```python
from build123d import *

# Parameters (mm, degrees)
SKETCH1_W                          = 200
SKETCH1_H                          = 90
BOSS_EXTRUDE1_DEPTH                = 40
SHAFTFITS_WITH_5MM_TOLERANCE_REACH = 120.743
SKETCH2_R                          = 3
SHAFTFITTOLERANCE_DEPTH            = 40
SKETCH3_R                          = 8.075
PULLEY_DEPTH                       = 30
SKETCH4_R                          = 26.5
GEARS_FITS_DEPTH                   = 10
GEAR_LETOUT_REACH                  = 120.743
SKETCH5_W                          = 200
SKETCH5_H                          = 30
CLOSED_LOOP_TIMING_BELT_REACH      = 116.891
SKETCH8_W                          = 60
SKETCH8_H                          = 3
SKETCH7_R                          = 10.075
PULLEY_MARGIN_DEPTH                = 20
SKETCH6_R                          = 28.5
GEAR_MARGIN_DEPTH                  = 10
PULLEYFIXTOLERANCE_DEPTH           = 30
GEARFITSTOLERANCE_DEPTH            = 10
M3_SCREWHOLES_REACH                = 116.891
M3_SCREWHEADS_DEPTH                = 5
M3_SCREWHEADS_DIRECTION_2_REACH    = 113.803
SKETCH16_W                         = 33
SKETCH16_H                         = 60
REMOVEEXTRA1_DEPTH                 = 40
SKETCH17_W                         = 5
SKETCH17_H                         = 60
REMOVEEXTRA2_DEPTH                 = 40


with BuildPart() as part:
    # Sketch1 → Boss-Extrude1 (new body)
    with BuildSketch(Plane.XY):
        with Locations((0, -5)):
            Rectangle(SKETCH1_W, SKETCH1_H)
    extrude(amount=BOSS_EXTRUDE1_DEPTH)

    # Sketch2 → ShaftFits_with.5mm_tolerance (cut, up to next)
    with BuildSketch(Plane.XY.offset(40), mode=Mode.PRIVATE) as shaftfits_with_5mm_tolerance_sk1:
        with Locations((30, 0)):
            Circle(SKETCH2_R)
    shaftfits_with_5mm_tolerance_tool1 = extrude(shaftfits_with_5mm_tolerance_sk1.sketch, amount=-SHAFTFITS_WITH_5MM_TOLERANCE_REACH, mode=Mode.PRIVATE) & part.part
    # Sketch2 → ShaftFits_with.5mm_tolerance (cut, up to next)
    with BuildSketch(Plane.XY.offset(40), mode=Mode.PRIVATE) as shaftfits_with_5mm_tolerance_sk2:
        with Locations(Location((-30, 0, 0), (0, 0, 180))):
            Circle(SKETCH2_R)
    shaftfits_with_5mm_tolerance_tool2 = extrude(shaftfits_with_5mm_tolerance_sk2.sketch, amount=-SHAFTFITS_WITH_5MM_TOLERANCE_REACH, mode=Mode.PRIVATE) & part.part
    add(shaftfits_with_5mm_tolerance_tool1.solids().sort_by_distance((30, 0, 40))[0], mode=Mode.SUBTRACT)
    add(shaftfits_with_5mm_tolerance_tool2.solids().sort_by_distance((-30, 0, 40))[0], mode=Mode.SUBTRACT)

    # Sketch9 → ShaftFitTolerance (cut)
    with BuildSketch(Plane.XY.offset(40)):
        with BuildLine():
            Line((30, 3), (35, 3))
            ThreePointArc((35, 3), (38, 0), (35, -3))
            Line((35, -3), (30, -3))
            ThreePointArc((30, -3), (27, 0), (30, 3))
        make_face()
    extrude(amount=-SHAFTFITTOLERANCE_DEPTH, mode=Mode.SUBTRACT)

    # Sketch3 → Pulley (cut)
    with BuildSketch(Plane.XY.offset(40)):
        with Locations((30, 0)):
            Circle(SKETCH3_R)
        with Locations(Location((-30, 0, 0), (0, 0, 180))):
            Circle(SKETCH3_R)
    extrude(amount=-PULLEY_DEPTH, mode=Mode.SUBTRACT)

    # Sketch4 → Gears fits (cut)
    with BuildSketch(Plane.XY.offset(40)):
        with Locations((30, 0)):
            Circle(SKETCH4_R)
        with Locations(Location((-30, 0, 0), (0, 0, 180))):
            Circle(SKETCH4_R)
    extrude(amount=-GEARS_FITS_DEPTH, mode=Mode.SUBTRACT)

    # Sketch5 → Gear letout (cut, up to next)
    with BuildSketch(Plane.XY.offset(40), mode=Mode.PRIVATE) as gear_letout_sk1:
        with Locations((0, -35)):
            Rectangle(SKETCH5_W, SKETCH5_H)
    gear_letout_tool1 = extrude(gear_letout_sk1.sketch, amount=-GEAR_LETOUT_REACH, mode=Mode.PRIVATE) & part.part
    add(gear_letout_tool1.solids().sort_by_distance((0, -35, 40))[0], mode=Mode.SUBTRACT)

    # Closed-loop timing belt: up to this face of the body (flat: up to its plane)
    closed_loop_timing_belt_end = Plane(part.part.faces().sort_by_distance((-22.15339549, 0, 10))[0])
    # Sketch8 → Closed-loop timing belt (cut, up to the picked face)
    with BuildSketch(Plane.XY.offset(40), mode=Mode.PRIVATE) as closed_loop_timing_belt_sk1:
        with Locations((0, 6.575)):
            Rectangle(SKETCH8_W, SKETCH8_H)
    closed_loop_timing_belt_tool1 = split(extrude(closed_loop_timing_belt_sk1.sketch, amount=-CLOSED_LOOP_TIMING_BELT_REACH, mode=Mode.PRIVATE), bisect_by=closed_loop_timing_belt_end, keep=Keep.BOTH, mode=Mode.PRIVATE)
    # Sketch8 → Closed-loop timing belt (cut, up to the picked face)
    with BuildSketch(Plane.XY.offset(40), mode=Mode.PRIVATE) as closed_loop_timing_belt_sk2:
        with Locations((0, -6.575)):
            Rectangle(SKETCH8_W, SKETCH8_H)
    closed_loop_timing_belt_tool2 = split(extrude(closed_loop_timing_belt_sk2.sketch, amount=-CLOSED_LOOP_TIMING_BELT_REACH, mode=Mode.PRIVATE), bisect_by=closed_loop_timing_belt_end, keep=Keep.BOTH, mode=Mode.PRIVATE)
    add(closed_loop_timing_belt_tool1.solids().sort_by(Axis((0, 6.575, 40), (0, 0, -1)))[0], mode=Mode.SUBTRACT)
    add(closed_loop_timing_belt_tool2.solids().sort_by(Axis((0, -6.575, 40), (0, 0, -1)))[0], mode=Mode.SUBTRACT)

    # Sketch7 → Pulley margin (cut)
    with BuildSketch(Plane.XY.offset(30)):
        with Locations((30, 0)):
            Circle(SKETCH7_R)
        with Locations((-30, 0)):
            Circle(SKETCH7_R)
    extrude(amount=-PULLEY_MARGIN_DEPTH, mode=Mode.SUBTRACT)

    # Sketch6 → Gear margin (cut)
    with BuildSketch(Plane.XY.offset(40)):
        with Locations((30, 0)):
            Circle(SKETCH6_R)
        with Locations((-30, 0)):
            Circle(SKETCH6_R)
    extrude(amount=-GEAR_MARGIN_DEPTH, mode=Mode.SUBTRACT)

    # Sketch12 → PulleyFixTolerance (cut)
    with BuildSketch(Plane.XY.offset(40)):
        with BuildLine():
            Line((30, 10.075), (35, 10.075))
            ThreePointArc((35, 10.075), (45.075, 0), (35, -10.075))
            Line((35, -10.075), (30, -10.075))
            ThreePointArc((30, -10.075), (19.925, 0), (30, 10.075))
        make_face()
    extrude(amount=-PULLEYFIXTOLERANCE_DEPTH, mode=Mode.SUBTRACT)

    # Sketch13 → GearFitsTolerance (cut)
    with BuildSketch(Plane.XY.offset(40)):
        with BuildLine():
            Line((30, 28.5), (35, 28.5))
            ThreePointArc((35, 28.5), (63.5, 0), (35, -28.5))
            Line((35, -28.5), (30, -28.5))
            ThreePointArc((30, -28.5), (1.5, 0), (30, 28.5))
        make_face()
    extrude(amount=-GEARFITSTOLERANCE_DEPTH, mode=Mode.SUBTRACT)

    # M3 ScrewHoles: up to this face of the body (flat: up to its plane)
    m3_screwholes_end = Plane(part.part.faces().sort_by_distance((0, -15.281996404, 40))[0])
    # Sketch14 → M3 ScrewHoles (cut, up to the picked face)
    with BuildSketch(Plane(origin=(0, 0, 0), x_dir=(-1, 0, 0), z_dir=(0, 0, -1)), mode=Mode.PRIVATE) as m3_screwholes_sk1:
        with BuildLine():
            Line((-6.5, 21.75), (-11.5, 21.75))
            ThreePointArc((-11.5, 21.75), (-13.25, 23.5), (-11.5, 25.25))
            Line((-11.5, 25.25), (-6.5, 25.25))
            ThreePointArc((-6.5, 25.25), (-4.75, 23.5), (-6.5, 21.75))
        make_face()
    m3_screwholes_tool1 = split(extrude(m3_screwholes_sk1.sketch, amount=-M3_SCREWHOLES_REACH, mode=Mode.PRIVATE), bisect_by=m3_screwholes_end, keep=Keep.BOTH, mode=Mode.PRIVATE)
    # Sketch14 → M3 ScrewHoles (cut, up to the picked face)
    with BuildSketch(Plane(origin=(0, 0, 0), x_dir=(-1, 0, 0), z_dir=(0, 0, -1)), mode=Mode.PRIVATE) as m3_screwholes_sk2:
        with BuildLine():
            Line((-53.5, 21.75), (-58.5, 21.75))
            ThreePointArc((-58.5, 21.75), (-60.25, 23.5), (-58.5, 25.25))
            Line((-58.5, 25.25), (-53.5, 25.25))
            ThreePointArc((-53.5, 25.25), (-51.75, 23.5), (-53.5, 21.75))
        make_face()
    m3_screwholes_tool2 = split(extrude(m3_screwholes_sk2.sketch, amount=-M3_SCREWHOLES_REACH, mode=Mode.PRIVATE), bisect_by=m3_screwholes_end, keep=Keep.BOTH, mode=Mode.PRIVATE)
    # Sketch14 → M3 ScrewHoles (cut, up to the picked face)
    with BuildSketch(Plane(origin=(0, 0, 0), x_dir=(-1, 0, 0), z_dir=(0, 0, -1)), mode=Mode.PRIVATE) as m3_screwholes_sk3:
        with BuildLine():
            Line((-53.5, -21.75), (-58.5, -21.75))
            ThreePointArc((-58.5, -21.75), (-60.25, -23.5), (-58.5, -25.25))
            Line((-58.5, -25.25), (-53.5, -25.25))
            ThreePointArc((-53.5, -25.25), (-51.75, -23.5), (-53.5, -21.75))
        make_face()
    m3_screwholes_tool3 = split(extrude(m3_screwholes_sk3.sketch, amount=-M3_SCREWHOLES_REACH, mode=Mode.PRIVATE), bisect_by=m3_screwholes_end, keep=Keep.BOTH, mode=Mode.PRIVATE)
    # Sketch14 → M3 ScrewHoles (cut, up to the picked face)
    with BuildSketch(Plane(origin=(0, 0, 0), x_dir=(-1, 0, 0), z_dir=(0, 0, -1)), mode=Mode.PRIVATE) as m3_screwholes_sk4:
        with BuildLine():
            Line((-6.5, -21.75), (-11.5, -21.75))
            ThreePointArc((-11.5, -21.75), (-13.25, -23.5), (-11.5, -25.25))
            Line((-11.5, -25.25), (-6.5, -25.25))
            ThreePointArc((-6.5, -25.25), (-4.75, -23.5), (-6.5, -21.75))
        make_face()
    m3_screwholes_tool4 = split(extrude(m3_screwholes_sk4.sketch, amount=-M3_SCREWHOLES_REACH, mode=Mode.PRIVATE), bisect_by=m3_screwholes_end, keep=Keep.BOTH, mode=Mode.PRIVATE)
    add(m3_screwholes_tool1.solids().sort_by(Axis((9, 23.5, 0), (0, 0, 1)))[0], mode=Mode.SUBTRACT)
    add(m3_screwholes_tool2.solids().sort_by(Axis((56, 23.5, 0), (0, 0, 1)))[0], mode=Mode.SUBTRACT)
    add(m3_screwholes_tool3.solids().sort_by(Axis((56, -23.5, 0), (0, 0, 1)))[0], mode=Mode.SUBTRACT)
    add(m3_screwholes_tool4.solids().sort_by(Axis((9, -23.5, 0), (0, 0, 1)))[0], mode=Mode.SUBTRACT)

    # Sketch15 → M3 ScrewHeads (cut)
    with BuildSketch(Plane.XY.offset(30)):
        with BuildLine():
            Line((6.5, 26.75), (11.5, 26.75))
            ThreePointArc((11.5, 26.75), (14.75, 23.5), (11.5, 20.25))
            Line((11.5, 20.25), (6.5, 20.25))
            ThreePointArc((6.5, 20.25), (3.25, 23.5), (6.5, 26.75))
        make_face()
        with BuildLine():
            Line((53.5, 26.75), (58.5, 26.75))
            ThreePointArc((58.5, 26.75), (61.75, 23.5), (58.5, 20.25))
            Line((58.5, 20.25), (53.5, 20.25))
            ThreePointArc((53.5, 20.25), (50.25, 23.5), (53.5, 26.75))
        make_face()
    extrude(amount=-M3_SCREWHEADS_DEPTH, mode=Mode.SUBTRACT)

    # M3 ScrewHeads direction 2: up to this face of the body (flat: up to its plane)
    m3_screwheads_direction_2_end = Plane(part.part.faces().sort_by_distance((0, -15.281996404, 40))[0])
    # Sketch15 → M3 ScrewHeads direction 2 (cut, up to the picked face)
    with BuildSketch(Plane.XY.offset(30), mode=Mode.PRIVATE) as m3_screwheads_direction_2_sk1:
        with BuildLine():
            Line((6.5, 26.75), (11.5, 26.75))
            ThreePointArc((11.5, 26.75), (14.75, 23.5), (11.5, 20.25))
            Line((11.5, 20.25), (6.5, 20.25))
            ThreePointArc((6.5, 20.25), (3.25, 23.5), (6.5, 26.75))
        make_face()
    m3_screwheads_direction_2_tool1 = split(extrude(m3_screwheads_direction_2_sk1.sketch, amount=M3_SCREWHEADS_DIRECTION_2_REACH, mode=Mode.PRIVATE), bisect_by=m3_screwheads_direction_2_end, keep=Keep.BOTH, mode=Mode.PRIVATE)
    # Sketch15 → M3 ScrewHeads direction 2 (cut, up to the picked face)
    with BuildSketch(Plane.XY.offset(30), mode=Mode.PRIVATE) as m3_screwheads_direction_2_sk2:
        with BuildLine():
            Line((53.5, 26.75), (58.5, 26.75))
            ThreePointArc((58.5, 26.75), (61.75, 23.5), (58.5, 20.25))
            Line((58.5, 20.25), (53.5, 20.25))
            ThreePointArc((53.5, 20.25), (50.25, 23.5), (53.5, 26.75))
        make_face()
    m3_screwheads_direction_2_tool2 = split(extrude(m3_screwheads_direction_2_sk2.sketch, amount=M3_SCREWHEADS_DIRECTION_2_REACH, mode=Mode.PRIVATE), bisect_by=m3_screwheads_direction_2_end, keep=Keep.BOTH, mode=Mode.PRIVATE)
    add(m3_screwheads_direction_2_tool1.solids().sort_by(Axis((9, 23.5, 30), (0, 0, 1)))[0], mode=Mode.SUBTRACT)
    add(m3_screwheads_direction_2_tool2.solids().sort_by(Axis((56, 23.5, 30), (0, 0, 1)))[0], mode=Mode.SUBTRACT)

    # Sketch16 → RemoveExtra1 (cut)
    with BuildSketch(Plane.XY.offset(40)):
        with Locations((-83.5, 10)):
            Rectangle(SKETCH16_W, SKETCH16_H)
        with Locations((83.5, 10)):
            Rectangle(SKETCH16_W, SKETCH16_H)
    extrude(amount=-REMOVEEXTRA1_DEPTH, mode=Mode.SUBTRACT)

    # Sketch17 → RemoveExtra2 (cut)
    with BuildSketch(Plane.XY.offset(40)):
        with Locations((-64.5, 10)):
            Rectangle(SKETCH17_W, SKETCH17_H)
    extrude(amount=-REMOVEEXTRA2_DEPTH, mode=Mode.SUBTRACT)


solid = part.part
```
Part model, mm, in its own coordinate system. A direction names the side the tool comes from. Round coordinates to 2 decimals unless told otherwise and drop trailing zeros. Write each loop counter-clockwise with the first axis right and the second up, starting at its lowest first coordinate (ties: lowest second). Pieces come first, ordered by that corner, then holes. Notation, with made-up numbers: M 1,31.5 L 23,31.5 A25 ccw 23,45.5 Z; hole C -30,-37.75 d6. An arc over 180 degrees is marked long. Answer as CSV lines item,"result". Start each with the question number.
1) Mould opens along X. For faces 1 (the face through (0, 5.075, 22)), 2 (the face through (2, 10, 0)), 3 (the face through (-62, 10, 20)) say: +X half, -X half, draft (parallel to the pull), parting line (faces both ways), or undercut.
2) Drill centre lines: L1, parallel to Y at x = -5.5, z = 16 (3 decimals); L2, parallel to X at y = 0, z = 33; L3, parallel to X at y = 0, z = 25 (3 decimals). Where is each one in solid material? Low to high.
3) Which spindle directions (+Z, -Z, +X, -X, +Y, -Y) get a long thin tool onto all of the face, cutting with end or side? Do faces 4 (the face through (60.25, 23.46, 12.32)), 5 (the face through (9, 21, 25)), 6 (the face through (67, 10, 20)). Say none if no direction does.
4) Band-saw the part on A-A (z = 12.5). List the corners of the cut face in (x, y) (3 decimals).
5) Band-saw the part on B-B (x = -30). List the corners of the cut face in (y, z) (3 decimals).
6) Drop a flat-ended pin along its axis: pin 1 (3 mm diameter, centred on x = 18.5, y = -1, fed in from +Z). Give the stop position or say it passes through.
7) Band-saw the part on C-C (y = 0). List the corners of the cut face in (x, z) (3 decimals), then the cut area to 3 significant figures.
8) Band-saw the part on D-D (z = 4). List the corners of the cut face in (x, y), then the cut area to 3 significant figures.
Worked out:
1,face 1,"undercut"
1,face 2,"draft"
1,face 3,"-X half"
2,L1,"-20 to -8.075, -5.075 to 5.075, 8.075 to 40"
2,L2,"-62 to -58.5, -1.5 to 1.5, 63.5 to 67"
2,L3,"-62 to -40.075, -19.925 to 19.925, 45.075 to 67"
3,face 4,"+Z, -Z"
3,face 5,"+Z"
3,face 6,"+Z, -Z, +X, +Y, -Y"
4,outline,"M -62,-20 L 67,-20 L 67,40 L -62,40 Z; M -21.297,-5.075 L 21.297,-5.075 A10.075 cw 21.297,5.075 L -21.297,5.075 A10.075 cw Z; hole M -23.975,-8.075 L 23.975,-8.075 A10.075 ccw 30,-10.075 L 35,-10.075 A10.075 ccw 35,10.075 L 30,10.075 A10.075 ccw 23.975,8.075 L -23.975,8.075 A10.075 ccw long Z; hole M 6.5,21.75 L 11.5,21.75 A1.75 ccw 11.5,25.25 L 6.5,25.25 A1.75 ccw Z; hole M 53.5,21.75 L 58.5,21.75 A1.75 ccw 58.5,25.25 L 53.5,25.25 A1.75 ccw Z"
5,outline,"M -20,0 L -3,0 L -3,10 L -10.075,10 L -10.075,30 L -20,30 Z; M 3,0 L 40,0 L 40,40 L 28.5,40 L 28.5,30 L 10.075,30 L 10.075,10 L 3,10 Z"
6,pin 1,"z = 30"
7,outline,"M -62,0 L -33,0 L -33,10 L -40.075,10 L -40.075,30 L -58.5,30 L -58.5,40 L -62,40 Z; M -27,0 L 27,0 L 27,10 L 19.925,10 L 19.925,30 L 1.5,30 L 1.5,40 L -1.5,40 L -1.5,30 L -19.925,30 L -19.925,10 L -27,10 Z; M 38,0 L 67,0 L 67,40 L 63.5,40 L 63.5,30 L 45.075,30 L 45.075,10 L 38,10 Z"
7,area,"2,890 mm²"
8,outline,"M -62,-20 L 67,-20 L 67,40 L -62,40 Z; hole C -30,0 d6; hole M 6.5,21.75 L 11.5,21.75 A1.75 ccw 11.5,25.25 L 6.5,25.25 A1.75 ccw Z; hole M 30,-3 L 35,-3 A3 ccw 35,3 L 30,3 A3 ccw Z; hole M 53.5,21.75 L 58.5,21.75 A1.75 ccw 58.5,25.25 L 53.5,25.25 A1.75 ccw Z"
8,area,"7,600 mm²"
